from build123d import *

# Parameters (mm, degrees)
F1_DEPTH  = 1.5875
F3_DEPTH  = 4.7625
F4_W      = 6.35
F4_H      = 6.35
F5_DEPTH  = 3.175
F6_SIZE   = 1.8598642
F7_W      = 28.575
F7_H      = 3.175
F8_DEPTH  = 1.5875
F9_W      = 25.4
F9_H      = 1.5875
F10_DEPTH = 6.35
F11_R     = 1.0922
F11_R_2   = 1.63322
F12_DEPTH = 25.4
F13_SIZE  = 1.58749
F14_R     = 0.396875
F15_DEPTH = 6.35
F16_R     = 1.63322
F17_DEPTH = 1.5875


# Not quite as in the source:
# - a fillet or chamfer is up to 0.001 mm smaller than in the source, because OpenCascade refuses the exact size


with BuildPart() as f1:
    # F0 (on Top) → F1 (new body)
    with BuildSketch(Plane.XY):
        Polygon((-87.87765, 22.225), (-127, 22.225), (-127, 17.4625), (-48.7553, 17.4625), (-26.5303, -4.7625), (26.5303, -4.7625), (48.7553, 17.4625), (127, 17.4625), (127, 22.225), (87.87765, 22.225), (46.7826079092, 45.9512336135), (-46.7826079092, 45.9512336135), align=None)
        Polygon((-24.5576079092, 0), (-46.7826079092, 22.225), (-78.35265, 22.225), (-45.5064998802, 41.1887336135), (45.5064998802, 41.1887336135), (78.35265, 22.225), (46.7826079092, 22.225), (24.5576079092, 0), align=None, mode=Mode.SUBTRACT)
    extrude(amount=F1_DEPTH)

    # F2 (on face) → F3 (join)
    with BuildSketch(Plane.XY.offset(1.5875)):
        Polygon((-127, 19.05), (-127, 17.4625), (-48.7553, 17.4625), (-26.5303, -4.7625), (26.5303, -4.7625), (48.7553, 17.4625), (127, 17.4625), (127, 19.05), (93.376911314, 19.05), (87.87765, 22.225), (46.7826079092, 45.9512336135), (-46.7826079092, 45.9512336135), (-87.87765, 22.225), (-93.376911314, 19.05), align=None)
        Polygon((90.201911314, 19.05), (48.0977359697, 19.05), (25.8727359697, -3.175), (14.2875, -3.175), (14.2875, -1.5875), (-14.2875, -1.5875), (-14.2875, -3.175), (-25.8727359697, -3.175), (-48.0977359697, 19.05), (-90.201911314, 19.05), (-46.3572385662, 44.3637336135), (-14.2875, 44.3637336135), (-14.2875, 42.7762336135), (14.2875, 42.7762336135), (14.2875, 44.3637336135), (46.3572385662, 44.3637336135), align=None, mode=Mode.SUBTRACT)
    extrude(amount=F3_DEPTH)

    # F4 (on face) → F5 (join, through all)
    with BuildSketch(Plane(origin=(0, 19.05, 0), x_dir=(-1, 0, 0), z_dir=(0, 1, 0))):
        with Locations((-53.5178, 3.175)):
            Rectangle(F4_W, F4_H)
        with Locations((-123.825, 3.175)):
            Rectangle(F4_W, F4_H)
        with Locations((123.825, 3.175)):
            Rectangle(F4_W, F4_H)
        with Locations((53.5178, 3.175)):
            Rectangle(F4_W, F4_H)
    extrude(amount=F5_DEPTH)

    # F6
    f6_edges = [f1.edges().sort_by_distance(p)[0] for p in [
        (-127, 19.84375, 6.35),
        (-120.65, 20.6375, 6.35),
        (-56.6928, 20.6375, 6.35),
        (-50.3428, 20.6375, 6.35),
        (50.3428, 20.6375, 6.35),
        (56.6928, 20.6375, 6.35),
        (120.65, 20.6375, 6.35),
        (127, 19.84375, 6.35),
    ]]
    chamfer(f6_edges, length=F6_SIZE)

    # F7 (on face) → F8 (join)
    with BuildSketch(Plane.XY.offset(6.35)):
        with Locations((0, -3.175)):
            Rectangle(F7_W, F7_H)
        with Locations((0, 44.3637336135)):
            Rectangle(F7_W, F7_H)
    extrude(amount=F8_DEPTH)

    # F9 (on face) → F10 (cut, through all)
    with BuildSketch(Plane.XY.offset(7.9375)):
        with Locations((0, -3.96875)):
            Rectangle(F9_W, F9_H)
        with Locations((0, 45.1574836135)):
            Rectangle(F9_W, F9_H)
    extrude(amount=-F10_DEPTH, mode=Mode.SUBTRACT)

    # F11 (on face) → F12 (cut, through all)
    with BuildSketch(Plane.XZ.offset(3.175)):
        with Locations((53.5178, 3.175)):
            Circle(F11_R)
        with Locations((123.825, 3.175)):
            Circle(F11_R)
        with Locations((-123.825, 3.175)):
            Circle(F11_R)
        with Locations((-53.5178, 3.175)):
            Circle(F11_R)
        with Locations((0, 4.7625)):
            Circle(F11_R_2)
    extrude(amount=-F12_DEPTH, mode=Mode.SUBTRACT)

    # F13 (size 1.5875 in the source; OpenCascade refuses exactly that, so slightly less here)
    f13_edges = [f1.edges().sort_by_distance(p)[0] for p in [
        (-14.2875, -3.96875, 6.35),
        (14.2875, -3.96875, 6.35),
        (-14.2875, 45.157484, 6.35),
        (14.2875, 45.157484, 6.35),
    ]]
    chamfer(f13_edges, length=F13_SIZE)

    # F14 (on face) → F15 (cut, through all)
    with BuildSketch(Plane.XY.offset(7.9375)):
        with Locations((-12.7, -3.175)):
            Circle(F14_R)
        with Locations((12.7, -3.175)):
            Circle(F14_R)
        with Locations((-12.7, 44.3637336135)):
            Circle(F14_R)
        with Locations((12.7, 44.3637336135)):
            Circle(F14_R)
    extrude(amount=-F15_DEPTH, mode=Mode.SUBTRACT)

    # F16 (on face) → F17 (cut, through all)
    with BuildSketch(Plane(origin=(0, 44.3637336135, 0), x_dir=(-1, 0, 0), z_dir=(0, 1, 0))):
        with Locations((0, 4.7625)):
            Circle(F16_R)
    extrude(amount=-F17_DEPTH, mode=Mode.SUBTRACT)


solid = f1.part
Part model, mm, in its own coordinate system. A direction names the side the tool comes from. Give positions to 0.01 mm unless a question says otherwise; leave off trailing zeros. Loops run counter-clockwise (first coordinate to the right, second up) from the corner with the lowest first, then second, coordinate; pieces in that order, holes last. Notation, with made-up numbers: M 61.5,17 L 72.5,17 A6 ccw 72.5,26 Z; hole C 82,-1.75 d2. An arc over 180 degrees is marked long. Put each result on its own line as item: value. Start each with the question number.
1) Flat gauge pins, fed straight in: pin 1 (2 mm diameter, centred on x = 0, z = 4.76, fed in from -Y); pin 2 (12 mm diameter, centred on x = 97, y = 20, fed in from +Z); pin 3 (1.9 mm diameter, centred on x = 95, z = 3, fed in from -Y); pin 4 (3 mm diameter, centred on x = -106, z = 2, fed in from +Y) (3 decimals). Where does each tip first touch, or does it go through?
2) Saw through at B-B (y = 15). List the corners of the cut face in (x, z).
3) Probe probe 1 along Z at (x, y) = (0, -1.95); probe 2 along Y at (x, z) = (-7, 6.5) (1 decimal); probe 3 along Y at (x, z) = (-68, 2). List the from-to ranges inside material, lowest first.
4) Pull direction Y, two halves, no side cores. Call faces 4 (the flat face through (66.2, 18.8, 6.35)), 5 (the flat face through (1, 45.951, 1)), 6 (the flat face through (-36.83, 7.78, 3.94)): +Y half, -Y half, draft (parallel to the pull), parting line (faces both ways), or undercut.
5) 3-axis set-ups, long thin cutter, end or side, ignore diameter. For faces 1 (the flat face through (20, -3.175, 4)), 2 (the flat face through (35.83, 11.27, 0.78)), 3 (the flat face through (-62.7, 18.8, 6.35)): which of +Z, -Z, +X, -X, +Y, -Y reach the whole face in a straight line?
Numbers:
1. pin 1: through
1. pin 2: z = 6.35
1. pin 3: y = 17.46
1. pin 4: y = 22.225
2. outline: M -46.29,0 L -39.56,0 L -39.56,1.59 L -44.05,1.59 L -44.05,6.35 L -46.29,6.35 Z; M 39.56,0 L 46.29,0 L 46.29,6.35 L 44.05,6.35 L 44.05,1.59 L 39.56,1.59 Z
3. probe 1: 0 to 3.13, 6.4 to 7.94
3. probe 2: -3.2 to -1.6, 42.8 to 44.4
3. probe 3: 17.46 to 19.05, 31.87 to 33.7
4. face 4: draft
4. face 5: +Y half
4. face 6: undercut
5. face 1: +Z
5. face 2: +Z, -Z
5. face 3: +Z, -X, +Y, -Y
